from build123d import *

# Parameters (mm, degrees)
ESQUISSE1_W                                   = 7
ESQUISSE1_H                                   = 8
BOSS_EXTRU_1_DEPTH                            = 40
TROU_POUR_TARAUDAGE_POUR_TROU_TARAUD_M3_D     = 2.5
TROU_POUR_TARAUDAGE_POUR_TROU_TARAUD_M3_DEPTH = 30
TROU_POUR_TARAUDAGE_POUR_TROU_TARAUD_M3_TIP   = 0.751075774
ESQUISSE4_R                                   = 1.6
ENL_V_MAT_EXTRU_1_DEPTH                       = 42.388404173


with BuildPart() as part:
    # Esquisse1 → Boss.-Extru.1 (new body)
    with BuildSketch(Plane.XY):
        with Locations((3.5, 4)):
            Rectangle(ESQUISSE1_W, ESQUISSE1_H)
    extrude(amount=BOSS_EXTRU_1_DEPTH)

    # Trou pour taraudage pour trou taraudé M31
    with Locations(Plane.XY.offset(40)):
        with Locations((3.5, 4)):
            Hole(TROU_POUR_TARAUDAGE_POUR_TROU_TARAUD_M3_D / 2, depth=TROU_POUR_TARAUDAGE_POUR_TROU_TARAUD_M3_DEPTH)
            with Locations((0, 0, -(TROU_POUR_TARAUDAGE_POUR_TROU_TARAUD_M3_DEPTH + TROU_POUR_TARAUDAGE_POUR_TROU_TARAUD_M3_TIP / 2))):  # 118° drill point
                Cone(0, TROU_POUR_TARAUDAGE_POUR_TROU_TARAUD_M3_D / 2, TROU_POUR_TARAUDAGE_POUR_TROU_TARAUD_M3_TIP, mode=Mode.SUBTRACT)

    # Esquisse4 → Enlèv. mat.-Extru.1 (cut, through all)
    with BuildSketch(Plane(origin=(0, 8, 0), x_dir=(1, 0, 0), z_dir=(0, 1, 0))):
        with Locations(Location((3.5, -5, 0), (0, 0, 270))):
            Circle(ESQUISSE4_R)
        with Locations(Location((3.5, -19, 0), (0, 0, 270))):
            Circle(ESQUISSE4_R)
    extrude(amount=-ENL_V_MAT_EXTRU_1_DEPTH, mode=Mode.SUBTRACT)


solid = part.part
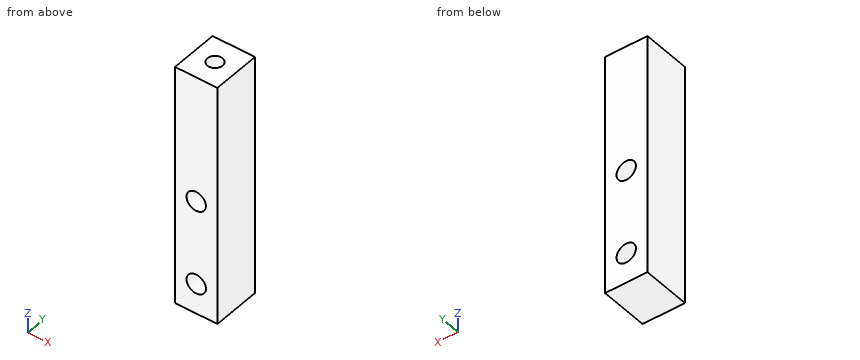
Build history of the part. All positions in model axes, mm. Coordinates: 2 decimals unless noted, no trailing zeros. Write each loop counter-clockwise with the first axis right and the second up, starting at its lowest first coordinate (ties: lowest second). Pieces come first, ordered by that corner, then holes.
(1) Drill centre lines: line 1 (Y direction, x = 3.5, z = 12.75); line 2 (X direction, y = 4.5, z = 19); line 3 (Z direction, x = 2.5, y = 7.5). Where is each one in solid material? Low to high.
(2) Cut at A-A on z = 5. List the corners of the cut face in (x, y), and give its area (3 significant figures).
(3) Pin check, flat tip, straight feed: pin 1 Ø1.9 at (x, z) = (3.5, 19) entering from -Y. Stop position of the tip, or through.
(4) Cut at B-B on z = 14. List the corners of the cut face in (x, y), and give its area (3 significant figures).
(5) Cut at C-C on y = 1.25. List the corners of the cut face in (x, z).
Working result:
1. line 1: y = 0 to 2.75, 5.25 to 8
1. line 2: x = 0 to 1.9, 5.1 to 7
1. line 3: z = 0 to 3.75, 6.25 to 17.75, 20.25 to 40
2. outline: (0, 0) - (1.9, 0) - (1.9, 8) - (0, 8) - close; (5.1, 0) - (7, 0) - (7, 8) - (5.1, 8) - close
2. area: 30.4 mm2
3. pin 1: passes through
4. outline: (0, 0) - (7, 0) - (7, 8) - (0, 8) - close; hole circle Ø2.5 at (3.5, 4)
4. area: 51.1 mm2
5. outline: (0, 0) - (7, 0) - (7, 40) - (0, 40) - close; hole circle Ø3.2 at (3.5, 5); hole circle Ø3.2 at (3.5, 19)
